Work out the finished part from the listing and answer in its coordinate system (mm). Face numbers are marked on the shaded views. A direction names the side the tool comes from. Coordinates: 2 decimals unless noted, no trailing zeros. Write each loop counter-clockwise with the first axis right and the second up, starting at its lowest first coordinate (ties: lowest second). Pieces come first, ordered by that corner, then holes. Notation, with made-up numbers: (-1, -11) - (31, -11) arc R21 ccw to (31, 12) - close; hole circle Ø10 at (73, 22.25). An arc over 180 degrees is marked (long way). Use one line per item in the form item = value. Start each with the question number.
Item 1: Determine the mould class of the marked faces 1, 2, 3 and 4 for opening direction X: released by +X, released by -X, zero draft, split by the parting line, or undercut.
Item 2: A cutting plane is placed at D-D (z = 28). Write down the section's boundary in (x, y), then the cut area to 3 significant figures.
Item 3: A cutting plane is placed at C-C (y = 5). Write down the section's boundary in (x, z).
Item 4: A cutting plane is placed at B-B (x = -70). Write down the section's boundary in (y, z), then the cut area to 3 significant figures.
Item 5: Given pin 1 (4 mm diameter, centred on x = -76, y = 4, fed in from -Z); pin 2 (5 mm diameter, centred on x = -76.5, z = -30, fed in from -Y), each flat-ended and moving along its own axis, determine where each tip first touches the part or whether it passes through.
Item 6: For the marked faces 5 and 6, determine the directions among +Z, -Z, +X, -X, +Y, -Y from which every point of the face is accessible in a straight line to the end or side of a thin tool.
Item 7: A cutting plane is placed at A-A (z = 9). Give the number of separate pieces and of enclosed holes in the cut face, then the cut area to 3 significant figures.
Item 8: Consider probe 1 along X at (y, z) = (2.5, 16); probe 2 along X at (y, z) = (0.5, -12); probe 3 along Z at (x, y) = (8, 1.5). Determine where each line is inside the solid, lowest interval first.
from build123d import *

# Parameters (mm, degrees)
EXTRUDE_1_DEPTH     = 42.5
SKETCH_2_OUTSIDE_W  = 135.498
SKETCH_2_OUTSIDE_H  = 57.498
CUT_EXTRUDE_1_DEPTH = 123
SKETCH_3_W          = 40
SKETCH_3_H          = 40
CUT_EXTRUDE_2_DEPTH = 8
SKETCH_4_W          = 223
SKETCH_4_H          = 82
CUT_EXTRUDE_3_DEPTH = 1
SKETCH_5_W          = 213
SKETCH_5_H          = 71
CUT_EXTRUDE_4_DEPTH = 1


with BuildPart() as part:
    # Эскиз1 → Бобышка-Вытянуть1 (new body, symmetric)
    with BuildSketch(Plane.XY):
        Polygon((-113.5, 0), (-113.5, 3.420983787), (-96.95384839, 7), (-46.95384839, 7), (-35.5, 3.420983787), (-24.04615161, 7), (24.04615161, 7), (35.5, 3.420983787), (46.95384839, 7), (96.95384839, 7), (113.5, 3.420983787), (113.5, 0), align=None)
    extrude(amount=EXTRUDE_1_DEPTH, both=True)

    # Эскиз2 outside → Вырез-Вытянуть1 (cut, symmetric)
    with BuildSketch(Plane(origin=(0, 0, 0), x_dir=(0, 0, -1), z_dir=(1, 0, 0))):
        with Locations((0, 3.5)):
            Rectangle(SKETCH_2_OUTSIDE_W, SKETCH_2_OUTSIDE_H)
        Polygon((42.5, 0), (-42.5, 0), (-42.5, 3.420983787), (-25, 7), (25, 7), (42.5, 3.420983787), align=None, mode=Mode.SUBTRACT)
    extrude(amount=CUT_EXTRUDE_1_DEPTH, both=True, mode=Mode.SUBTRACT)

    # Эскиз3 → Вырез-Вытянуть2 (cut, through all)
    with BuildSketch(Plane.XZ):
        with Locations((71, 0)):
            Rectangle(SKETCH_3_W, SKETCH_3_H)
        Rectangle(SKETCH_3_W, SKETCH_3_H)
        with Locations((-71, 0)):
            Rectangle(SKETCH_3_W, SKETCH_3_H)
    extrude(amount=-CUT_EXTRUDE_2_DEPTH, mode=Mode.SUBTRACT)

    # Эскиз4 → Вырез-Вытянуть3 (cut)
    with BuildSketch(Plane.XZ):
        Rectangle(SKETCH_4_W, SKETCH_4_H)
    extrude(amount=-CUT_EXTRUDE_3_DEPTH, mode=Mode.SUBTRACT)

    # Эскиз5 → Вырез-Вытянуть4 (cut)
    with BuildSketch(Plane.XZ.offset(-1)):
        Rectangle(SKETCH_5_W, SKETCH_5_H)
    extrude(amount=-CUT_EXTRUDE_4_DEPTH, mode=Mode.SUBTRACT)


solid = part.part
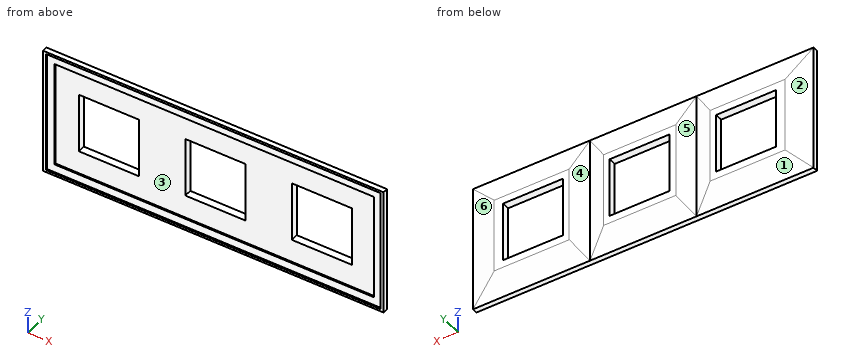
Answer:
q1.face_1 = zero draft
q1.face_2 = released by -X
q1.face_3 = undercut
q1.face_4 = undercut
q2.outline = (-113.5, 0) - (-111.5, 0) - (-111.5, 1) - (-106.5, 1) - (-106.5, 2) - (106.5, 2) - (106.5, 1) - (111.5, 1) - (111.5, 0) - (113.5, 0) - (113.5, 3.42) - (99.79, 6.39) - (44.99, 6.39) - (35.5, 3.42) - (26.01, 6.39) - (-26.01, 6.39) - (-35.5, 3.42) - (-44.99, 6.39) - (-99.79, 6.39) - (-113.5, 3.42) - close
q2.area = 917 mm²
q3.outline = (-106.2, -34.78) - (-40.55, -34.78) - (-40.55, 34.78) - (-106.2, 34.78) - close; (-30.45, -34.78) - (30.45, -34.78) - (30.45, 34.78) - (-30.45, 34.78) - close; (40.55, -34.78) - (106.2, -34.78) - (106.2, 34.78) - (40.55, 34.78) - close; hole (-91, -20) - (-51, -20) - (-51, 20) - (-91, 20) - close; hole (-20, -20) - (20, -20) - (20, 20) - (-20, 20) - close; hole (51, -20) - (91, -20) - (91, 20) - (51, 20) - close
q4.outline = (0, -42.5) - (3.42, -42.5) - (7, -25) - (7, -20) - (2, -20) - (2, -35.5) - (1, -35.5) - (1, -41) - (0, -41) - close; (0, 41) - (1, 41) - (1, 35.5) - (2, 35.5) - (2, 20) - (7, 20) - (7, 25) - (3.42, 42.5) - (0, 42.5) - close
q4.area = 179 mm²
q5.pin_1 = -42.5
q5.pin_2 = 2
q6.face_5 = +Z, -Z, +Y
q6.face_6 = +Z, -Z, +X, +Y
q7.separate_pieces = 4
q7.enclosed_holes = 0
q7.area = 412 mm²
q8.probe_1 = -113.5 to -91, -51 to -20, 20 to 51, 91 to 113.5
q8.probe_2 = -113.5 to -111.5, 111.5 to 113.5
q8.probe_3 = -42.5 to -35.5, 35.5 to 42.5
